from build123d import *

# Parameters (mm, degrees)
SKETCH1_R                = 13.5
SKETCH1_R_2              = 1.8288
SKETCH1_R_3              = 11.1125
SKETCH1_R_4              = 2.65
BOSS_EXTRUDE1_DEPTH      = 3.175
CUT_EXTRUDE1_REACH       = 179.004
SKETCH2_W                = 4.112404804
SKETCH2_H                = 127.6975
FILLET3_R                = 2.5
FILLET4_R                = 25
M2_5X0_45_TAPPED_HOLE1_D = 2.05
F_6_CLEARANCE_HOLE1_D    = 3.7973


with BuildPart() as part:
    # Sketch1 → Boss-Extrude1 (new body)
    with BuildSketch(Plane(origin=(0, 0, 0), x_dir=(0, 0, -1), z_dir=(1, 0, 0))):
        with BuildLine():
            Line((20.757404804, -103.81), (20.757404804, -5))
            Line((20.757404804, -5), (16.645, 5.681808734))
            Line((16.645, 5.681808734), (16.645, 35))
            ThreePointArc((16.645, 35), (14.175569213, 43.724062271), (7.5, 49.85954323))
            Line((7.5, 49.85954323), (7.5, 116.469314765))
            ThreePointArc((7.5, 116.469314765), (0, 174.5), (-7.5, 116.469314765))
            Line((-7.5, 116.469314765), (-7.5, 49.85954323))
            ThreePointArc((-7.5, 49.85954323), (-14.175569213, 43.724062271), (-16.645, 35))
            Line((-16.645, 35), (-16.645, 5.681808734))
            Line((-16.645, 5.681808734), (-20.757404804, -5))
            Line((-20.757404804, -5), (-20.757404804, -103.81))
            Line((-20.757404804, -103.81), (20.757404804, -103.81))
        make_face()
        with Locations((0, 145)):
            Circle(SKETCH1_R, mode=Mode.SUBTRACT)
        with Locations((-13.4747, -100)):
            Circle(SKETCH1_R_2, mode=Mode.SUBTRACT)
        with Locations((13.4747, -100)):
            Circle(SKETCH1_R_2, mode=Mode.SUBTRACT)
        with Locations((-13.4747, 0)):
            Circle(SKETCH1_R_2, mode=Mode.SUBTRACT)
        with Locations((13.4747, 0)):
            Circle(SKETCH1_R_2, mode=Mode.SUBTRACT)
        with Locations((0, 35)):
            Circle(SKETCH1_R_3, mode=Mode.SUBTRACT)
        with Locations((18.619546181, 134.25)):
            Circle(SKETCH1_R_4, mode=Mode.SUBTRACT)
        with Locations((0, 166.5)):
            Circle(SKETCH1_R_4, mode=Mode.SUBTRACT)
        with Locations((-18.619546181, 134.25)):
            Circle(SKETCH1_R_4, mode=Mode.SUBTRACT)
    extrude(amount=BOSS_EXTRUDE1_DEPTH)

    # Sketch2 → Cut-Extrude1 (cut, up to next)
    with BuildSketch(Plane(origin=(3.175, 0, 0), x_dir=(0, 0, -1), z_dir=(1, 0, 0)), mode=Mode.PRIVATE) as cut_extrude1_sk1:
        Polygon((11.645, -5), (-11.645, -5), (11.645, -27.976379872), align=None)
    cut_extrude1_tool1 = extrude(cut_extrude1_sk1.sketch, amount=-CUT_EXTRUDE1_REACH, mode=Mode.PRIVATE) & part.part
    # Sketch2 → Cut-Extrude1 (cut, up to next)
    with BuildSketch(Plane(origin=(3.175, 0, 0), x_dir=(0, 0, -1), z_dir=(1, 0, 0)), mode=Mode.PRIVATE) as cut_extrude1_sk2:
        Polygon((-11.645, -12.023620128), (11.645, -35), (-11.645, -57.976379872), (-11.645, -35), align=None)
    cut_extrude1_tool2 = extrude(cut_extrude1_sk2.sketch, amount=-CUT_EXTRUDE1_REACH, mode=Mode.PRIVATE) & part.part
    # Sketch2 → Cut-Extrude1 (cut, up to next)
    with BuildSketch(Plane(origin=(3.175, 0, 0), x_dir=(0, 0, -1), z_dir=(1, 0, 0)), mode=Mode.PRIVATE) as cut_extrude1_sk3:
        Polygon((-11.645, -72.023620128), (-11.645, -95), (11.645, -95), align=None)
    cut_extrude1_tool3 = extrude(cut_extrude1_sk3.sketch, amount=-CUT_EXTRUDE1_REACH, mode=Mode.PRIVATE) & part.part
    # Sketch2 → Cut-Extrude1 (cut, up to next)
    with BuildSketch(Plane(origin=(3.175, 0, 0), x_dir=(0, 0, -1), z_dir=(1, 0, 0)), mode=Mode.PRIVATE) as cut_extrude1_sk4:
        Polygon((11.645, -42.023620128), (11.645, -65), (11.645, -87.976379872), (-11.645, -65), align=None)
    cut_extrude1_tool4 = extrude(cut_extrude1_sk4.sketch, amount=-CUT_EXTRUDE1_REACH, mode=Mode.PRIVATE) & part.part
    # Sketch2 → Cut-Extrude1 (cut, up to next)
    with BuildSketch(Plane(origin=(3.175, 0, 0), x_dir=(0, 0, -1), z_dir=(1, 0, 0)), mode=Mode.PRIVATE) as cut_extrude1_sk5:
        with Locations((-18.701202402, -39.96125)):
            Rectangle(SKETCH2_W, SKETCH2_H)
    cut_extrude1_tool5 = extrude(cut_extrude1_sk5.sketch, amount=-CUT_EXTRUDE1_REACH, mode=Mode.PRIVATE) & part.part
    # Sketch2 → Cut-Extrude1 (cut, up to next)
    with BuildSketch(Plane(origin=(3.175, 0, 0), x_dir=(0, 0, -1), z_dir=(1, 0, 0)), mode=Mode.PRIVATE) as cut_extrude1_sk6:
        with Locations((18.701202402, -39.96125)):
            Rectangle(SKETCH2_W, SKETCH2_H)
    cut_extrude1_tool6 = extrude(cut_extrude1_sk6.sketch, amount=-CUT_EXTRUDE1_REACH, mode=Mode.PRIVATE) & part.part
    add(cut_extrude1_tool1.solids().sort_by_distance((3.175, -12.658793, -3.881667))[0], mode=Mode.SUBTRACT)
    add(cut_extrude1_tool2.solids().sort_by_distance((3.175, -35, 3.881667))[0], mode=Mode.SUBTRACT)
    add(cut_extrude1_tool3.solids().sort_by_distance((3.175, -87.341207, 3.881667))[0], mode=Mode.SUBTRACT)
    add(cut_extrude1_tool4.solids().sort_by_distance((3.175, -65, -3.881667))[0], mode=Mode.SUBTRACT)
    add(cut_extrude1_tool5.solids().sort_by_distance((3.175, -39.96125, 18.701202))[0], mode=Mode.SUBTRACT)
    add(cut_extrude1_tool6.solids().sort_by_distance((3.175, -39.96125, -18.701202))[0], mode=Mode.SUBTRACT)

    # Fillet3
    fillet3_edges = [part.edges().sort_by_distance(p)[0] for p in [
        (1.5875, -103.81, 16.645),
        (1.5875, -12.023620128, 11.645),
        (1.5875, -35, -11.645),
        (1.5875, -57.976379872, 11.645),
        (1.5875, -103.81, -16.645),
        (1.5875, -72.023620128, 11.645),
        (1.5875, -95, -11.645),
        (1.5875, -95, 11.645),
        (1.5875, -87.976379872, -11.645),
        (1.5875, -65, 11.645),
        (1.5875, -42.023620128, -11.645),
        (1.5875, -27.976379872, -11.645),
        (1.5875, -5, 11.645),
        (1.5875, -5, -11.645),
    ]]
    fillet(fillet3_edges, radius=FILLET3_R)

    # Fillet4
    fillet4_edges = [part.edges().sort_by_distance(p)[0] for p in [
        (1.5875, 49.85954323, 7.5),
        (1.5875, 116.469314765, 7.5),
        (1.5875, 116.469314765, -7.5),
        (1.5875, 49.85954323, -7.5),
    ]]
    fillet(fillet4_edges, radius=FILLET4_R)

    # M2.5x0.45 Tapped Hole1 (through all)
    with Locations(Plane(origin=(3.175, 0, 0), x_dir=(0, 0, -1), z_dir=(1, 0, 0))):
        with Locations((23.015, 145), (-23.015, 145)):
            Hole(M2_5X0_45_TAPPED_HOLE1_D / 2)

    # #6 Clearance Hole1 (through all)
    with Locations(Plane(origin=(3.175, 0, 0), x_dir=(0, 0, -1), z_dir=(1, 0, 0))):
        with Locations((0, 90)):
            Hole(F_6_CLEARANCE_HOLE1_D / 2)


solid = part.part
The model under review builds one solid part; all positions refer to its coordinate system, in mm. A direction names the side the tool comes from. Coordinates: 2 decimals unless noted, no trailing zeros. Order: outer loops, then holes, each group sorted by start corner. A loop starts at its lowest first (then second) coordinate and runs counter-clockwise, first axis right, second up. Notation, with made-up numbers: (-32, -38) -> (23, -38) arc R24 cw to (23, -25) -> close; hole circle Ø9 at (13, -26). An arc over 180 degrees is marked (long way). Answer in a Markdown table with one row per item.
(1) Wall thickness on line 1 along Z through (x, y) = (1.4, -100) (1 decimal); line 2 along Z through (x, y) = (1, 90); line 3 along Y through (x, z) = (1.05, -12): over which ranges is each line inside the solid? List them lowest first.
Answers:
| item | result |
|---|---|
| line 1 | -16.6 to -15.3, -11.6 to 11.6, 15.3 to 16.6 |
| line 2 | -7.5 to -1.9, 1.9 to 7.5 |
| line 3 | -103.81 to -101.08, -98.92 to -1.08, 1.08 to 46.73, 115.56 to 138.82, 151.18 to 171.95 |
(2) The part is to be moulded in two halves that separate along Y. For faces 4 (the flat face through (3.175, 68, 0)), 5 (the cylindrical face through (1.565, 174.482, -1.033)), 6 (the flat face through (1.61, -24.602, -1.105)), say which applies: +Y half, -Y half, draft (parallel to the pull), parting line (faces both ways), or undercut.
Answers:
| item | result |
|---|---|
| face 4 | draft |
| face 5 | parting line |
| face 6 | undercut |
(3) Insertion check: pin 1 (1 mm diameter, centred on x = 2.5, y = -38.5, fed in from -Z) (3 decimals); pin 2 (3.5 mm diameter, centred on y = 90, z = 0, fed in from +X); pin 3 (1 mm diameter, centred on x = 1, y = 82, fed in from -Z); pin 4 (6 mm diameter, centred on y = 113.5, z = -8.5, fed in from -X). Each pin has a flat end and moves straight along its axis. Give the tip position at first contact, or say it passes through.
Answers:
| item | result |
|---|---|
| pin 1 | z = -16.645 |
| pin 2 | through |
| pin 3 | z = -7.5 |
| pin 4 | x = 0 |
(4) Consider section D-D (y = 63.5). Write out the cut boundary in (x, z) (3 decimals).
Answers:
| item | result |
|---|---|
| outline | (0, -7.5) -> (3.175, -7.5) -> (3.175, 7.5) -> (0, 7.5) -> close |
(5) Consider section A-A (y = -41). Write out the cut boundary in (x, z) (3 decimals).
Answers:
| item | result |
|---|---|
| outline | (0, -16.645) -> (3.175, -16.645) -> (3.175, -5.563) -> (0, -5.563) -> close; (0, 11.645) -> (3.175, 11.645) -> (3.175, 16.645) -> (0, 16.645) -> close |
(6) Consider section B-B (y = 134.25). Write out the cut boundary in (x, z) (3 decimals), plus the area to 3 significant figures.
Answers:
| item | result |
|---|---|
| outline | (0, -27.472) -> (3.175, -27.472) -> (3.175, -21.27) -> (0, -21.27) -> close; (0, -15.97) -> (3.175, -15.97) -> (3.175, -8.166) -> (0, -8.166) -> close; (0, 8.166) -> (3.175, 8.166) -> (3.175, 15.97) -> (0, 15.97) -> close; (0, 21.27) -> (3.175, 21.27) -> (3.175, 27.472) -> (0, 27.472) -> close |
| area | 88.9 mm² |
(7) Consider section C-C (x = 1.35). State how many separate pieces and enclosed holes the cut face has, plus the area to 3 significant figures.
Answers:
| item | result |
|---|---|
| separate pieces | 1 |
| enclosed holes | 16 |
| area | 6,220 mm² |
(8) Machinability: for faces 1 (the cylindrical face through (1.61, 112.63, -10.24)), 2 (the flat face through (1.61, -16.43, 0.06)), 3 (the cylindrical face through (1.61, 112.336, 10.092)), which of the approach directions +Z, -Z, +X, -X, +Y, -Y give a long, thin tool a straight path to every point of the face, cutting with its end or side? Answer none if there is none.
Answers:
| item | result |
|---|---|
| face 1 | -Z, +X, -X |
| face 2 | +X, -X |
| face 3 | +Z, +X, -X |
